Read the model definition and answer for the solid it produces. Units are mm, in the model's axes. Coordinates: 2 decimals unless noted, no trailing zeros. Write each loop counter-clockwise with the first axis right and the second up, starting at its lowest first coordinate (ties: lowest second). Pieces come first, ordered by that corner, then holes. Notation, with made-up numbers: M 69.5,-37 L 102.5,-37 A20 cw 102.5,-24 Z; hole C 45.25,-19.75 d5. An arc over 180 degrees is marked long. Use a Markdown table: item, result. Add a question column.
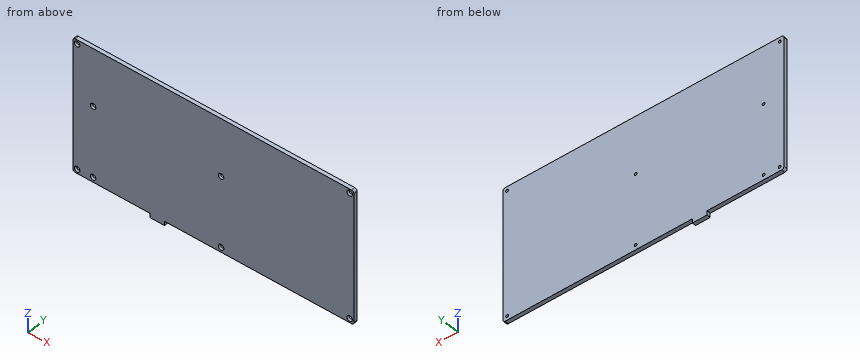
from build123d import *

# Parameters (mm, degrees)
SALIENTE_EXTRUIR1_DEPTH                              = 2.5
REDONDEO1_R                                          = 1.5
CSK_FOR_M1_6_COUNTERSUNK_FLAT_HEAD_SCREW_D           = 1.8
CSK_FOR_M1_6_COUNTERSUNK_FLAT_HEAD_SCREW_CSINK_D     = 3.6
CSK_FOR_M1_6_COUNTERSUNK_FLAT_HEAD_SCREW_CSINK_ANGLE = 90


with BuildPart() as part:
    # Croquis1 → Saliente-Extruir1 (new body)
    with BuildSketch(Plane(origin=(0, 0, 0), x_dir=(1, 0, 0), z_dir=(0, 1, 0))):
        Polygon((-90.389050604, -43.256388366), (94.110949396, -43.256388366), (94.110949396, 43.657904704), (-30.269137665, 43.657904704), (-30.269137665, 46.407904704), (-39.909137665, 46.407904704), (-39.909137665, 43.657904704), (-90.389050604, 43.657904704), align=None)
    extrude(amount=SALIENTE_EXTRUIR1_DEPTH)

    # Redondeo1
    redondeo1_edges = [part.edges().sort_by_distance(p)[0] for p in [
        (-90.389050604, 1.25, 43.256388366),
        (-90.389050604, 1.25, -43.657904704),
        (94.110949396, 1.25, -43.657904704),
        (94.110949396, 1.25, 43.256388366),
    ]]
    fillet(redondeo1_edges, radius=REDONDEO1_R)

    # CSK for M1.6 Countersunk Flat Head Screw1 (through all)
    with Locations(Plane(origin=(-87.639050604, 0, 40.506388366), x_dir=(0, 0, -1), z_dir=(0, -1, 0))):
        with Locations((0, 0), (0, 179), (81.41429307, 179), (81.41429307, 0), (34.81029307, 10.55), (34.81029307, 94.55), (80.91429307, 94.55), (80.91429307, 10.55)):
            CounterSinkHole(CSK_FOR_M1_6_COUNTERSUNK_FLAT_HEAD_SCREW_D / 2, CSK_FOR_M1_6_COUNTERSUNK_FLAT_HEAD_SCREW_CSINK_D / 2, counter_sink_angle=CSK_FOR_M1_6_COUNTERSUNK_FLAT_HEAD_SCREW_CSINK_ANGLE)


solid = part.part
Item 1: Each of these flat-tipped pins is pushed along its axis until it touches: pin 1 (1.2 mm diameter, centred on y = 2, z = -45.5, fed in from -X); pin 2 (1.6 mm diameter, centred on x = 91.36, z = 40.51, fed in from -Y); pin 3 (1.2 mm diameter, centred on y = 1, z = -45.5, fed in from +X); pin 4 (1.2 mm diameter, centred on x = 23.5, y = 1, fed in from -Z). Where does it stop, or does it pass through?
Item 2: Consider probe 1 along X at (y, z) = (0.85, -41.5); probe 2 along Z at (x, y) = (55, 1.95). Determine where each line is inside the solid, lowest interval first.
Item 3: Find section B-B on x = -57. Give the vertices of the cut face in (y, z), then the cut area to 3 significant figures.
Item 4: Find section A-A on y = 1.45. Count the separate pieces of the cut face and the enclosed holes in it, then the cut area to 3 significant figures.
Geometry says:
| question | item | result |
|---|---|---|
| 1 | pin 1 | stops at x = -39.91 |
| 1 | pin 2 | passes through |
| 1 | pin 3 | stops at x = -30.27 |
| 1 | pin 4 | stops at z = -43.66 |
| 2 | probe 1 | x = -90.39 to -88.38, -86.9 to 90.62, 92.1 to 94.11 |
| 2 | probe 2 | z = -43.66 to 43.26 |
| 3 | outline | M 0,-43.66 L 2.5,-43.66 L 2.5,43.26 L 0,43.26 Z |
| 3 | area | 217 mm2 |
| 4 | separate pieces | 1 |
| 4 | enclosed holes | 8 |
| 4 | area | 16,000 mm2 |
